The model under review builds one solid part; all positions refer to its coordinate system, in mm. Face numbers are marked on the shaded views. A direction names the side the tool comes from. Give positions to 0.01 mm unless a question says otherwise; leave off trailing zeros. Loops run counter-clockwise (first coordinate to the right, second up) from the corner with the lowest first, then second, coordinate; pieces in that order, holes last. Notation, with made-up numbers: M 43.25,81.5 L 95.25,81.5 A17 cw 95.25,110.5 Z; hole C 30.25,33.5 d5. An arc over 180 degrees is marked long. Return JSON: item names as keys, results as strings.
Autodesk Inventor part; units mm, degrees
ref_plane "b_XY" through (-4.953, 4.7625, 0) normal (0, 0, 1) x (1, 0, 0)
ref_plane "b_YZ" through (-4.953, 4.7625, 0) normal (1, 0, 0) x (0, 1, 0)
ref_plane "b_ZX" through (-4.953, 4.7625, 0) normal (0, 1, 0) x (0, 0, 1)
sketch "Sketch_1" plane through (0, 0, 0) normal (0, 0, 1) x (1, 0, 0)
  line L0 (4.953, 0) -> (-4.953, 0)
  line L1 (-5.5626, 7.4168) -> (-5.5626, 5.3721)
  arc A0 (-5.5626, 5.3721) -> (-4.953, 4.7625) centre (-4.953, 5.3721) ccw
  line L2 (-4.953, 4.7625) -> (4.953, 4.7625)
  arc A1 (4.953, 4.7625) -> (5.5626, 5.3721) centre (4.953, 5.3721) ccw
  line L3 (5.5626, 5.3721) -> (5.5626, 7.4168)
  line L4 (5.5626, 7.4168) -> (5.4483, 7.4168)
  line L5 (5.4483, 7.4168) -> (5.4483, 7.3025)
  line L6 (5.4483, 7.3025) -> (5.334, 7.3025)
  line L7 (5.334, 7.3025) -> (5.334, 10.1727)
  line L8 (5.334, 10.1727) -> (5.4483, 10.1727)
  line L9 (5.4483, 10.1727) -> (5.4483, 10.0584)
  line L10 (5.4483, 10.0584) -> (5.5626, 10.0584)
  line L11 (5.5626, 10.0584) -> (5.5626, 12.7)
  line L12 (5.5626, 12.7) -> (2.8956, 15.367)
  line L13 (2.8956, 15.367) -> (2.667, 15.367)
  line L14 (2.667, 15.367) -> (0.7112, 13.4112)
  line L15 (0.7112, 13.4112) -> (0.7112, 12.7)
  arc A2 (-0.7112, 12.7) -> (0.7112, 12.7) centre (0, 12.7) ccw
  line L16 (-0.7112, 12.7) -> (-0.7112, 13.4112)
  line L17 (-0.7112, 13.4112) -> (-2.667, 15.367)
  line L18 (-2.667, 15.367) -> (-2.8956, 15.367)
  line L19 (-2.8956, 15.367) -> (-5.5626, 12.7)
  line L20 (-5.5626, 12.7) -> (-5.5626, 10.0584)
  line L21 (-5.5626, 10.0584) -> (-5.4483, 10.0584)
  line L22 (-5.4483, 10.0584) -> (-5.4483, 10.1727)
  line L23 (-5.4483, 10.1727) -> (-5.334, 10.1727)
  line L24 (-5.334, 10.1727) -> (-5.334, 7.3025)
  line L25 (-5.334, 7.3025) -> (-5.4483, 7.3025)
  line L26 (-5.4483, 7.3025) -> (-5.4483, 7.4168)
  line L27 (-5.4483, 7.4168) -> (-5.5626, 7.4168)
revolve "Revolution1" add sketch "Sketch_1" angle 360 about axis through (4.953, 0, 0) along (1, 0, 0)
ref_plane "b_XY" through (-4.953, 4.7625, 0) normal (0, 0, 1) x (1, 0, 0)
ref_plane "b_YZ" through (-4.953, 4.7625, 0) normal (1, 0, 0) x (0, 1, 0)
ref_plane "b_ZX" through (-4.953, 4.7625, 0) normal (0, 1, 0) x (0, 0, 1)
ref_plane "b1_XY" through (-4.953, -4.7625, 0) normal (0, 0, 1) x (1, 0, 0)
ref_plane "b1_YZ" through (-4.953, -4.7625, 0) normal (1, 0, 0) x (0, 1, 0)
ref_plane "b1_ZX" through (-4.953, -4.7625, 0) normal (0, 1, 0) x (0, 0, 1)
ref_plane "d_XY" through (-2.7813, 15.367, 0) normal (0, 0, 1) x (1, 0, 0)
ref_plane "d_YZ" through (-2.7813, 15.367, 0) normal (1, 0, 0) x (0, 1, 0)
ref_plane "d_ZX" through (-2.7813, 15.367, 0) normal (0, 1, 0) x (0, 0, 1)
ref_plane "d1_XY" through (-2.7813, -15.367, 0) normal (0, 0, 1) x (1, 0, 0)
ref_plane "d1_YZ" through (-2.7813, -15.367, 0) normal (1, 0, 0) x (0, 1, 0)
ref_plane "d1_ZX" through (-2.7813, -15.367, 0) normal (0, 1, 0) x (0, 0, 1)
ref_plane "vri_XY" through (0, 12.7, 0) normal (0, 0, 1) x (1, 0, 0)
ref_plane "vri_YZ" through (0, 12.7, 0) normal (1, 0, 0) x (0, 1, 0)
ref_plane "vri_ZX" through (0, 12.7, 0) normal (0, 1, 0) x (0, 0, 1)
ref_plane "vri1_XY" through (5.5626, 0, 0) normal (0, 0, 1) x (1, 0, 0)
ref_plane "vri1_YZ" through (5.5626, 0, 0) normal (1, 0, 0) x (0, 1, 0)
ref_plane "vri1_ZX" through (5.5626, 0, 0) normal (0, 1, 0) x (0, 0, 1)
ref_plane "w_XY" through (-5.5626, 12.7, 0) normal (0, 0, 1) x (1, 0, 0)
ref_plane "w_YZ" through (-5.5626, 12.7, 0) normal (1, 0, 0) x (0, 1, 0)
ref_plane "w_ZX" through (-5.5626, 12.7, 0) normal (0, 1, 0) x (0, 0, 1)
ref_plane "w1_XY" through (5.5626, 12.7, 0) normal (0, 0, 1) x (1, 0, 0)
ref_plane "w1_YZ" through (5.5626, 12.7, 0) normal (1, 0, 0) x (0, 1, 0)
ref_plane "w1_ZX" through (5.5626, 12.7, 0) normal (0, 1, 0) x (0, 0, 1)
ref_plane "wheel_XY" through (5.5626, 0, 0) normal (1, 0, 0) x (0, 0, -1)
ref_plane "wheel_YZ" through (5.5626, 0, 0) normal (0, 0, -1) x (0, 1, 0)
ref_plane "wheel_ZX" through (5.5626, 0, 0) normal (0, 1, 0) x (1, 0, 0)
ref_plane "wheel2_XY" through (-5.5626, 0, 0) normal (1, 0, 0) x (0, 0, -1)
ref_plane "wheel2_YZ" through (-5.5626, 0, 0) normal (0, 0, -1) x (0, 1, 0)
ref_plane "wheel2_ZX" through (-5.5626, 0, 0) normal (0, 1, 0) x (1, 0, 0)
properties part number "W2X"
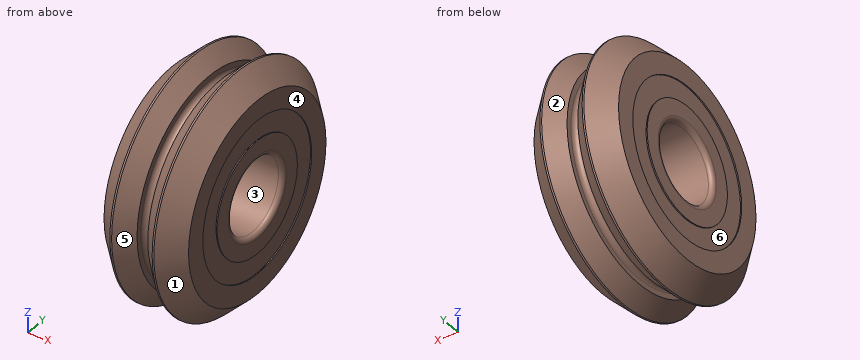
1) Consider section B-B on x = 4. Write out the cut boundary in (y, z) (1 decimal), then the cut area to 3 significant figures.
From the geometry:
{"outline": "C 0,0 d28.5; hole C 0,0 d9.5", "area": "568 mm²"}
2) Tool access review of the marked faces 1 and 2: name each direction out of +Z, -Z, +X, -X, +Y, -Y from which nothing blocks a thin tool from reaching the whole face with its end or side.
From the geometry:
{"face 1": "+X", "face 2": "none"}
3) Wall thickness on L1, parallel to Z at x = -4.5, y = -1; L2, parallel to X at y = 2, z = -8; L3, parallel to X at y = -5, z = 12.5: over which ranges is each line inside the solid? List them lowest first. Write a range as from..to.
From the geometry:
{"L1": "-13.73..-4.66, 4.66..13.73", "L2": "-5.33..5.33", "L3": "-4.8..-0.76, 0.76..4.8"}
4) Insertion check: pin 1 (1 mm diameter, centred on y = 8, z = -4, fed in from -X); pin 2 (1.5 mm diameter, centred on x = -1, z = -11.5, fed in from -Y); pin 3 (1.5 mm diameter, centred on x = 2.5, y = -6.5, fed in from +Z). Each pin has a flat end and moves straight along its axis. Give the tip position at first contact, or say it passes through.
From the geometry:
{"pin 1": "x = -5.33", "pin 2": "y = -9.08", "pin 3": "z = 14.24"}
5) Consider section A-A on x = -2. Write out the cut boundary in (y, z) (1 decimal).
From the geometry:
{"outline": "C 0,0 d29.4; hole C 0,0 d9.5"}
6) The part is to be moulded in two halves that separate along Y. For the marked faces 3, 4, 5 and 6, say which applies: released by +Y, released by -Y, zero draft, split by the parting line, or undercut.
From the geometry:
{"face 3": "undercut", "face 4": "zero draft", "face 5": "split by the parting line", "face 6": "undercut"}
